Geometry check sheet. Reference: the model listing, model coordinates, mm. A direction names the side the tool comes from. Give positions to 0.01 mm unless a question says otherwise; leave off trailing zeros. Write each loop counter-clockwise with the first axis right and the second up, starting at its lowest first coordinate (ties: lowest second). Pieces come first, ordered by that corner, then holes. Notation, with made-up numbers: (88, 77) -> (113, 77) arc R22 cw to (113, 88) -> close; hole circle Ø2 at (-35.5, 36). An arc over 180 degrees is marked (long way). Write item = value, one per line. Start each with the question number.
1. Cross-section at B-B, the plane x = 0. Record the cut outline in (y, z) (3 decimals), plus the area to 3 significant figures.
2. Thickness scan on line 1 along X through (y, z) = (2, 0); line 2 along X through (y, z) = (12.25, 0.5) (3 decimals); line 3 along Y through (x, z) = (-1, 4.75) (3 decimals). Record the ranges inside material, lowest first.
3. Depth check by flat-ended pin: P1, Ø2.5, axis at x = 0, z = 6, coming from the -Y side; P2, Ø3, axis at x = -15, z = 0, coming from the -Y side; P3, Ø3, axis at x = -14, z = -0.5, coming from the +Y side. Enter the tip coordinate at first touch or a pass-through.
4. Cross-section at C-C, the plane y = 3.75. Record the cut outline in (x, z).
5. Cross-section at D-D, the plane z = 3. Record the cut outline in (x, y), plus the area to 3 significant figures.
6. Set-up check for faces 1 (the cylindrical face through (-0.26, 11.483, -1.423)), 2 (the flat face through (-2.72, 7.96, 5.52)), 3 (the flat face through (-13.46, 14.07, 2.72)): record each of +Z, -Z, +X, -X, +Y, -Y from which the full face is reachable in a straight line by a thin tool's end or side.
7. Mould release check, pull along X, two halves, no side actions. Record for faces 4 (the flat face through (20, 9, 0)), 5 (the flat face through (0, 7, -7)), 6 (the flat face through (-5, 16, 0)): pulls with the +X half, pulls with the -X half, needs draft (parallel to the pull), parting line crosses it, or undercut.
8. Cross-section at A-A, the plane z = 0. State how many separate pieces and enclosed holes the cut face has, plus the area to 3 significant figures.
```python
from build123d import *

# Parameters (mm, degrees)
SKETCH1_W           = 40
SKETCH1_H           = 14
BOSS_EXTRUDE1_DEPTH = 19
SKETCH2_W           = 10
SKETCH2_H           = 3
SKETCH2_H_2         = 1
CUT_EXTRUDE1_DEPTH  = 30
SKETCH3_R           = 2
CUT_EXTRUDE2_DEPTH  = 31.935416597
SKETCH4_R           = 1.6
CUT_EXTRUDE3_DEPTH  = 29.460498942
CUT_EXTRUDE4_DEPTH  = 10
CUT_EXTRUDE5_DEPTH  = 3


with BuildPart() as part:
    # Sketch1 → Boss-Extrude1 (new body)
    with BuildSketch(Plane(origin=(0, 0, 0), x_dir=(1, 0, 0), z_dir=(0, 1, 0))):
        Rectangle(SKETCH1_W, SKETCH1_H)
    extrude(amount=BOSS_EXTRUDE1_DEPTH)

    # Sketch2 → Cut-Extrude1 (cut)
    with BuildSketch(Plane.XY.offset(7)):
        with Locations((0, 16)):
            Rectangle(SKETCH2_W, SKETCH2_H)
        Rectangle(SKETCH2_W, SKETCH2_H_2)
    extrude(amount=-CUT_EXTRUDE1_DEPTH, mode=Mode.SUBTRACT)

    # Sketch3 → Cut-Extrude2 (cut, through all)
    with BuildSketch(Plane.XY.offset(7)):
        with Locations((0, 9.5)):
            Circle(SKETCH3_R)
    extrude(amount=-CUT_EXTRUDE2_DEPTH, mode=Mode.SUBTRACT)

    # Sketch4 → Cut-Extrude3 (cut, through all)
    with BuildSketch(Plane(origin=(0, 19, 0), x_dir=(1, 0, 0), z_dir=(0, 1, 0))):
        with Locations(Location((-15, 0, 0), (0, 0, 270))):
            Circle(SKETCH4_R)
        with Locations(Location((15, 0, 0), (0, 0, 90))):
            Circle(SKETCH4_R)
    extrude(amount=-CUT_EXTRUDE3_DEPTH, mode=Mode.SUBTRACT)

    # Sketch9 → Cut-Extrude4 (cut)
    with BuildSketch(Plane(origin=(0, 19, 0), x_dir=(1, 0, 0), z_dir=(0, 1, 0))):
        Polygon((-15, 3.608439182), (-18.125, 1.804219591), (-18.125, -1.804219591), (-15, -3.608439182), (-11.875, -1.804219591), (-11.875, 1.804219591), align=None)
        Polygon((11.875, 1.804219591), (15, 3.608439182), (18.125, 1.804219591), (18.125, -1.804219591), (15, -3.608439182), (11.875, -1.804219591), align=None)
    extrude(amount=-CUT_EXTRUDE4_DEPTH, mode=Mode.SUBTRACT)

    # Sketch10 → Cut-Extrude5 (cut)
    with BuildSketch(Plane.XY.offset(7)):
        Polygon((1.804219591, 12.625), (-1.804219591, 12.625), (-3.608439182, 9.5), (-1.804219591, 6.375), (1.804219591, 6.375), (3.608439182, 9.5), align=None)
    extrude(amount=-CUT_EXTRUDE5_DEPTH, mode=Mode.SUBTRACT)


solid = part.part
```
Answers:
q1.outline = (0.5, -7) -> (7.5, -7) -> (7.5, 4) -> (6.375, 4) -> (6.375, 7) -> (0.5, 7) -> close; (11.5, -7) -> (14.5, -7) -> (14.5, 7) -> (12.625, 7) -> (12.625, 4) -> (11.5, 4) -> close; (17.5, -7) -> (19, -7) -> (19, 7) -> (17.5, 7) -> close
q1.area = 154 mm^2
q2.line_1 = -20 to -16.6, -13.4 to 13.4, 16.6 to 20
q2.line_2 = -20 to -18.125, -11.875 to 11.875, 18.125 to 20
q2.line_3 = 0.5 to 6.375, 12.625 to 14.5, 17.5 to 19
q3.P1 = 0.5
q3.P2 = through
q3.P3 = 9
q4.outline = (-20, -7) -> (20, -7) -> (20, 7) -> (-20, 7) -> close; hole circle Ø3.2 at (-15, 0); hole circle Ø3.2 at (15, 0)
q5.outline = (-20, 0) -> (-5, 0) -> (-5, 0.5) -> (5, 0.5) -> (5, 0) -> (20, 0) -> (20, 19) -> (16.05, 19) -> (16.05, 9) -> (13.95, 9) -> (13.95, 19) -> (-13.95, 19) -> (-13.95, 9) -> (-16.05, 9) -> (-16.05, 19) -> (-20, 19) -> close; hole (-5, 14.5) -> (5, 14.5) -> (5, 17.5) -> (-5, 17.5) -> close; hole circle Ø4 at (0, 9.5)
q5.area = 670 mm^2
q6.face_1 = +Z, -Z
q6.face_2 = +Z
q6.face_3 = +Y
q7.face_4 = pulls with the +X half
q7.face_5 = needs draft
q7.face_6 = undercut
q8.separate_pieces = 3
q8.enclosed_holes = 2
q8.area = 530 mm^2
